Autodesk Inventor part; units mm, degrees
ref_plane "YZ Plane" through (0, 0, 0) normal (1, 0, 0) x (0, 1, 0)
ref_plane "XZ Plane" through (0, 0, 0) normal (0, 1, 0) x (-1, 0, 0)
ref_plane "XY Plane" through (0, 0, 0) normal (0, 0, 1) x (1, 0, 0)
sketch "Sketch1" plane through (0, 0, 0) normal (0, 1, 0) x (-1, 0, 0)
  line L0 (3, 9) -> (-3, 9)
  line L1 (-3, 9) -> (-3, -9)
  line L2 (-3, -9) -> (3, -9)
  line L3 (3, -9) -> (3, 9)
  line L4 (3, 9) -> (-3, -9) construction
  line L5 (-3, 9) -> (3, -9) construction
  circle A0 centre (0, 9) radius 3
  circle A1 centre (0, -9) radius 3
  line L6 (-3, -9) -> (-7, -9)
  line L7 (-7, -9) -> (-7, -5)
  line L8 (-7, -5) -> (-7, -3)
  line L9 (-7, -3) -> (-3, -3)
  line L10 (-7, -3) -> (-7, -6)
  circle A2 centre (-7, -6) radius 3
  line L11 (-3, -3) -> (-3, -9)
  point P0 (0, 0)
  dimension "d0" = 6
  dimension "d1" = 18
  dimension "d2" = 6
  dimension "d4" = 6
  dimension "d5" = 4
  dimension "d6" = 4
  dimension "d7" = 2
  dimension "d10" = 3
  dimension "d11" = 6
extrude "Extrusion1" add sketch "Sketch1" along normal blind 1.5 contours A0 L0 | L0 A0 | L3 A1 L1 A0 | A1 L2 | L2 A1 | A2 L7 L8 | L8 L7 A2
sketch "Sketch2" plane through (0, 1.5, 0) normal (0, 1, 0) x (1, 0, 0)
  line L0 (3, -9) -> (3, 9)
  arc A0 (3, 9) -> (-3, 9) centre (0, 9) ccw
  line L1 (-3, 9) -> (-3, -9)
  arc A1 (-3, -9) -> (3, -9) centre (0, -9) ccw
  circle A2 centre (0, 9) radius 1.5
  circle A3 centre (0, -9) radius 1.5
  line L2 (3, 9) -> (7, 9)
  line L3 (7, 9) -> (7, 3)
  line L4 (7, 3) -> (3, 3)
  line L5 (3, 3) -> (3, 9)
  point P0 (0, 0)
  dimension "d14" = 3
  dimension "d15" = 3
  dimension "d16" = 4
  dimension "d17" = 6
extrude "Extrusion2" cut sketch "Sketch2" against normal blind 1.5 contours L0 L2 L3 L4 | A2 | A3
sketch "Sketch3" plane through (0, 1.5, 0) normal (0, 1, 0) x (1, 0, 0)
  line L0 (3, -9) -> (3, 9)
  arc A0 (3, 9) -> (-3, 9) centre (0, 9) ccw
  line L1 (-3, 9) -> (-3, -9)
  line L2 (3, 9) -> (7, 9)
  line L3 (7, 9) -> (7, 3)
  line L4 (7, 3) -> (3, 3)
  line L5 (3, 3) -> (3, 9)
  point P0 (0, 0)
  dimension "d20" = 4
  dimension "d21" = 6
  dimension "d22" = 4
extrude "Extrusion3" add sketch "Sketch3" against normal blind 1.5
sketch "Sketch4" plane through (0, 1.5, 0) normal (0, 1, 0) x (1, 0, 0)
  arc A0 (7, 3) -> (7, 9) centre (7, 6) ccw
  circle A1 centre (7, 6) radius 1.5
  point P0 (0, 0)
  dimension "d25" = 3
extrude "Extrusion4" cut sketch "Sketch4" against normal blind 1.5
sketch "Sketch5" plane through (0, 0, 0) normal (0, -1, 0) x (1, 0, 0)
  circle A0 centre (7, -6) radius 1.5
  circle A1 centre (0, 9) radius 1.5
  circle A2 centre (0, -9) radius 1.5
  arc A3 (7, -9) -> (7, -3) centre (7, -6) ccw
  arc A4 (3, 9) -> (-3, 9) centre (0, 9) ccw
  arc A5 (-3, -9) -> (3, -9) centre (0, -9) ccw
  circle A6 centre (0, 9) radius 0.1
  circle A7 centre (0, -9) radius 0.1
  circle A8 centre (7, -6) radius 0.1
  point P0 (0, 0)
  dimension "d28" = 0.2
  dimension "d29" = 0.2
  dimension "d30" = 0.2
extrude "Extrusion5" add sketch "Sketch5" against normal blind 1.5
sketch "Sketch6" plane through (0, 0, 0) normal (0, -1, 0) x (1, 0, 0)
  circle A0 centre (0, -9) radius 0.1
  circle A1 centre (7, -6) radius 0.1
  circle A2 centre (0, 9) radius 0.1
  arc A3 (7, -9) -> (7, -3) centre (7, -6) ccw
  arc A4 (3, 9) -> (-3, 9) centre (0, 9) ccw
  arc A5 (-3, -9) -> (3, -9) centre (0, -9) ccw
  circle A6 centre (0, 9) radius 1.5
  circle A7 centre (0, -9) radius 1.5
  circle A8 centre (7, -6) radius 1.5
  point P0 (0, 0)
  dimension "d33" = 3
  dimension "d34" = 3
  dimension "d35" = 3
extrude "Extrusion6" cut sketch "Sketch6" against normal blind 2
sketch "Sketch7" plane through (0, 0, 0) normal (0, -1, 0) x (1, 0, 0)
  arc A0 (-3, -9) -> (3, -9) centre (0, -9) ccw
  line L0 (3, -9) -> (7, -9)
  line L1 (0, -9) -> (0, -5)
  circle A1 centre (0, -5) radius 1.5
  point P0 (0, 0)
  dimension "d38" = 4
  dimension "d39" = 3
extrude "Extrusion7" cut sketch "Sketch7" against normal blind 2
sketch "Sketch8" plane through (0, 0, 0) normal (0, -1, 0) x (1, 0, 0)
  circle A0 centre (0, -5) radius 1.5
  point P0 (0, 0)
extrude "Extrusion8" add sketch "Sketch8" against normal blind 2
sketch "Sketch9" plane through (0, 2, -5) normal (0, 1, 0) x (1, 0, 0)
  circle A0 centre (0, 0) radius 1.5
  point P0 (0, -5)
extrude "Extrusion9" cut sketch "Sketch9" against normal blind 0.5
properties part number "tahlo3"
Could you check a few things on this model? Use its own coordinates, in mm. A direction names the side the tool comes from. Give positions to 0.01 mm unless a question says otherwise; leave off trailing zeros. Loops run counter-clockwise (first coordinate to the right, second up) from the corner with the lowest first, then second, coordinate; pieces in that order, holes last. Notation, with made-up numbers: (56.5, -20.5) - (67.5, -20.5) arc R8 ccw to (67.5, -11.5) - close; hole circle Ø8 at (20.5, 79). An arc over 180 degrees is marked (long way). Answer in a Markdown table with one row per item. Add a question column.
Q1. If we section it at D-D (x = 1.25): List the corners of the cut face in (y, z) for me.
Q2. If we section it at B-B (x = -0.75): List the corners of the cut face in (y, z) for me.
Q3. If we section it at C-C (y = 0.75): List the corners of the cut face in (x, z) for me.
Q4. If we section it at A-A (z = -6): List the corners of the cut face in (x, y) for me, plus the area to 3 significant figures.
Q5. Please list where these lines run through material, in increasing order: L1, parallel to Z at x = 0, y = 0.5; L2, parallel to Z at x = 7, y = 0.9; L3, parallel to Z at x = -0.75, y = 0.65. Write a range as from..to.
Q6. We'd pull the mould along X, two halves only. Please class faces 4 (the face through (10, 1, -6)), 5 (the face through (5.5, 0.74, -5.93)), 6 (the face through (-3, 1, 0)): +X half, -X half, draft (parallel to the pull), parting line (faces both ways), or undercut.
Q7. Which directions (+Z, -Z, +X, -X, +Y, -Y) give clear straight access to the entire face, cutting with the end or side of a thin tool? Please do faces 1 (the face through (0, 1, -12)), 2 (the face through (5, 1, -9)), 3 (the face through (3, 1, 3)).
Q8. For pin 1 (0.8 mm diameter, centred on x = 4.5, y = 1, fed in from -Z); pin 2 (0.8 mm diameter, centred on y = 0.5, z = 1.5, fed in from +X), each with a flat end and sliding along its axis, tell me the tip position at first contact or that it passes through.
The answers:
| question | item | result |
|---|---|---|
| 1 | outline | (0, -11.73) - (1.5, -11.73) - (1.5, -9.83) - (0, -9.83) - close; (0, -8.17) - (1.5, -8.17) - (1.5, 8.17) - (0, 8.17) - close; (0, 9.83) - (1.5, 9.83) - (1.5, 11.73) - (0, 11.73) - close |
| 2 | outline | (0, -11.9) - (1.5, -11.9) - (1.5, -10.3) - (0, -10.3) - close; (0, -7.7) - (1.5, -7.7) - (1.5, 7.7) - (0, 7.7) - close; (0, 10.3) - (1.5, 10.3) - (1.5, 11.9) - (0, 11.9) - close |
| 3 | outline | (-3, -9) arc R3 ccw to (3, -9) - (7, -9) arc R3 ccw to (7, -3) - (3, -3) - (3, 9) arc R3 ccw to (-3, 9) - close; hole circle Ø3 at (0, -9); hole circle Ø3 at (0, 9); hole circle Ø3 at (7, -6) |
| 4 | outline | (-3, 0) - (5.5, 0) - (5.5, 1.5) - (-3, 1.5) - close; (8.5, 0) - (10, 0) - (10, 1.5) - (8.5, 1.5) - close |
| 4 | area | 15.0 mm^2 |
| 5 | L1 | z = -12..-10.5, -7.5..7.5, 10.5..12 |
| 5 | L2 | z = -9..-7.5, -4.5..-3 |
| 5 | L3 | z = -11.9..-10.3, -7.7..7.7, 10.3..11.9 |
| 6 | face 4 | +X half |
| 6 | face 5 | undercut |
| 6 | face 6 | -X half |
| 7 | face 1 | -Z, +Y, -Y |
| 7 | face 2 | -Z, +X, +Y, -Y |
| 7 | face 3 | +Z, +X, +Y, -Y |
| 8 | pin 1 | stops at z = -9 |
| 8 | pin 2 | stops at x = 3 |
